```python
from build123d import *

# Parameters (mm, degrees)
F1_DEPTH = 25


with BuildPart() as f1:
    # F0 (on Top) → F1 (new body)
    with BuildSketch(Plane.XY):
        with BuildLine():
            Line((121.561594, 52.757246), (-104.438406, 52.757246))
            Line((-104.438406, 52.757246), (-104.438406, 26.757246))
            Line((-104.438406, 26.757246), (-17.188406, 26.757246))
            ThreePointArc((-17.188406, 26.757246), (-4.460484, 21.485168), (0.811594, 8.757246))
            Line((0.811594, 8.757246), (0.811594, -143.248167))
            ThreePointArc((0.811594, -143.248167), (-4.460484, -155.976089), (-17.188406, -161.248167))
            Line((-17.188406, -161.248167), (-103.907911, -161.248167))
            Line((-103.907911, -161.248167), (-104.438406, -187.242754))
            Line((-104.438406, -187.242754), (109.092089, -187.242754))
            Line((109.092089, -187.242754), (109.092089, -161.248167))
            Line((109.092089, -161.248167), (34.311594, -161.248167))
            ThreePointArc((34.311594, -161.248167), (21.583672, -155.976089), (16.311594, -143.248167))
            Line((16.311594, -143.248167), (16.311594, 8.757246))
            ThreePointArc((16.311594, 8.757246), (21.583672, 21.485168), (34.311594, 26.757246))
            Line((34.311594, 26.757246), (121.561594, 26.757246))
            Line((121.561594, 26.757246), (121.561594, 52.757246))
        make_face()
    extrude(amount=F1_DEPTH)


solid = f1.part
```
Build history of the part. All positions in model axes, mm. A direction names the side the tool comes from. Round coordinates to 2 decimals unless told otherwise and drop trailing zeros. Write each loop counter-clockwise with the first axis right and the second up, starting at its lowest first coordinate (ties: lowest second). Pieces come first, ordered by that corner, then holes.
1) Band-saw the part on C-C, the plane y = -37. List the corners of the cut face in (x, z), and give its area (4 significant figures).
2) Band-saw the part on D-D, the plane y = 21.5. List the corners of the cut face in (x, z).
3) Mould opens along Y. For faces 4 (the flat face through (8, -67, 25)), 5 (the flat face through (0.812, -66, 12)), 6 (the flat face through (10, 52.757, 12)) say: +Y half, -Y half, draft (parallel to the pull), parting line (faces both ways), or undercut.
4) Band-saw the part on B-B, the plane z = 5.25. List the corners of the cut face in (x, y).
5) Band-saw the part on A-A, the plane x = 77.5. List the corners of the cut face in (y, z), and give its area (3 significant figures).
6) 3-axis set-ups, long thin cutter, end or side, ignore diameter. For faces 1 (the cylindrical face through (21.724, -156.115, 12.325)), 2 (the flat face through (-60, -161.248, 12)), 3 (the flat face through (109.092, -174, 12)): which of +Z, -Z, +X, -X, +Y, -Y reach the whole face in a straight line?
7) Pin check, flat tips, straight feed: pin 1 (12.5 mm diameter, centred on y = -35.5, z = 13, fed in from -X); pin 2 (12.5 mm diameter, centred on y = -51.5, z = 7, fed in from +X). Stop position of each tip, or through.
8) Drill centre lines: probe 1 along Y at (x, z) = (-38, 16.5); probe 2 along X at (y, z) = (-129, 21.5); probe 3 along X at (y, z) = (-146, 1.5). Where is each one in solid material? Low to high.
Ans:
1. outline: (0.81, 0) - (16.31, 0) - (16.31, 25) - (0.81, 25) - close
1. area: 387.5 mm2
2. outline: (-4.48, 0) - (21.6, 0) - (21.6, 25) - (-4.48, 25) - close
3. face 4: draft
3. face 5: undercut
3. face 6: +Y half
4. outline: (-104.44, -187.24) - (109.09, -187.24) - (109.09, -161.25) - (34.31, -161.25) arc R18 cw to (16.31, -143.25) - (16.31, 8.76) arc R18 cw to (34.31, 26.76) - (121.56, 26.76) - (121.56, 52.76) - (-104.44, 52.76) - (-104.44, 26.76) - (-17.19, 26.76) arc R18 cw to (0.81, 8.76) - (0.81, -143.25) arc R18 cw to (-17.19, -161.25) - (-103.91, -161.25) - close
5. outline: (-187.24, 0) - (-161.25, 0) - (-161.25, 25) - (-187.24, 25) - close; (26.76, 0) - (52.76, 0) - (52.76, 25) - (26.76, 25) - close
5. area: 1,300 mm2
6. face 1: +Z, -Z, +X
6. face 2: +Z, -Z, -X
6. face 3: +Z, -Z, +X, -Y
7. pin 1: stops at x = 0.81
7. pin 2: stops at x = 16.31
8. probe 1: y = -187.24 to -161.25, 26.76 to 52.76
8. probe 2: x = 0.81 to 16.31
8. probe 3: x = 0.6 to 16.52
